Work out the finished part from the listing and answer in its coordinate system (mm). Face numbers are marked on the shaded views. Coordinates: 2 decimals unless noted, no trailing zeros. Loops run counter-clockwise (first coordinate to the right, second up) from the corner with the lowest first, then second, coordinate; pieces in that order, holes last. Notation, with made-up numbers: (-29, 45) - (24, 45) arc R29 cw to (24, 81) - close; hole circle Ø11 at (-4.5, -33). An arc over 180 degrees is marked (long way). Write each question's results on one line, items separated by ' | '. Start each with the question number.
Item 1: Section C-C, the plane x = 2.35 is taken. Write down the section's boundary in (y, z), plus the area to 3 significant figures.
Item 2: Consider probe 1 along Y at (x, z) = (0, 1.6); probe 2 along Z at (x, y) = (-0.2, -1.9); probe 3 along X at (y, z) = (0.2, 3.75). Determine where each line is inside the solid, lowest interval first. Write a range as [from, to].
Item 3: Section A-A, the plane z = 11.25 is taken. Write down the section's boundary in (x, y), plus the area to 3 significant figures.
Item 4: This flat-tipped pin is pushed along its axis until it touches: pin 1 Ø1.5 at (x, y) = (1.5, 0) entering from -Z. Where does it stop, or does it pass through?
Item 5: Section B-B, the plane y = -1.85 is taken. Write down the section's boundary in (x, z), plus the area to 3 significant figures.
Item 6: For a pull along Y with two mould halves and no side action, classify the marked faces 1, 2, 3 and 4 as +Y half, -Y half, draft (parallel to the pull), parting line (faces both ways), or undercut.
Item 7: Section D-D, the plane z = 22.5 is taken. Write down the section's boundary in (x, y), plus the area to 3 significant figures.
from build123d import *

# Parameters (mm, degrees)
EXTRUDE_1_DEPTH = 20
SKETCH_2_R      = 1.5
EXTRUDE_2_DEPTH = 4
M3X0_5_1_D      = 2.5
M3X0_5_1_DEPTH  = 5
M3X0_5_1_TIP    = 0.751075774


with BuildPart() as part:
    # 草圖1 → 填料-伸長1 (new body)
    with BuildSketch(Plane.XY):
        Polygon((2.70199926, 0), (1.35099963, 2.34), (-1.35099963, 2.34), (-2.70199926, 0), (-1.35099963, -2.34), (1.35099963, -2.34), align=None)
    extrude(amount=EXTRUDE_1_DEPTH)

    # 草圖2 → 填料-伸長2 (add)
    with BuildSketch(Plane.XY.offset(20)):
        Circle(SKETCH_2_R)
    extrude(amount=EXTRUDE_2_DEPTH)

    # M3x0.5 螺紋孔1
    with Locations(Plane(origin=(0, 0, 0), x_dir=(-1, 0, 0), z_dir=(0, 0, -1))):
        with Locations((0, 0)):
            Hole(M3X0_5_1_D / 2, depth=M3X0_5_1_DEPTH)
            with Locations((0, 0, -(M3X0_5_1_DEPTH + M3X0_5_1_TIP / 2))):  # 118° drill point
                Cone(0, M3X0_5_1_D / 2, M3X0_5_1_TIP, mode=Mode.SUBTRACT)


solid = part.part
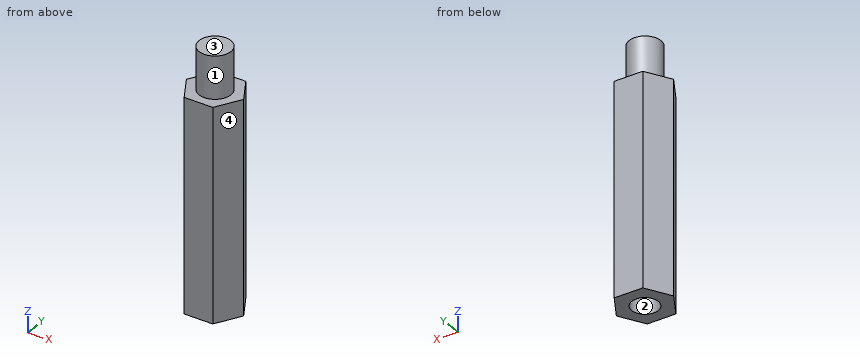
Answer key:
1) outline: (-0.61, 0) - (0.61, 0) - (0.61, 20) - (-0.61, 20) - close | area: 24.4 mm^2
2) probe 1: y = [-2.34, -1.25], [1.25, 2.34] | probe 2: z = [0, 20] | probe 3: x = [-2.59, -1.23], [1.23, 2.59]
3) outline: (-2.7, 0) - (-1.35, -2.34) - (1.35, -2.34) - (2.7, 0) - (1.35, 2.34) - (-1.35, 2.34) - close | area: 19.0 mm^2
4) pin 1: stops at z = 0
5) outline: (-1.63, 0) - (1.63, 0) - (1.63, 20) - (-1.63, 20) - close | area: 65.4 mm^2
6) face 1: parting line | face 2: undercut | face 3: draft | face 4: -Y half
7) outline: circle Ø3 at (0, 0) | area: 7.07 mm^2
